from build123d import *

# Parameters (mm, degrees)
SKETCH_1_W               = 80
SKETCH_1_H               = 80
EXTRUDE_1_DEPTH          = 20
SKETCH_2_R               = 15
CUT_EXTRUDE_1_DEPTH      = 20
SKETCH_3_R               = 2
CUT_EXTRUDE_2_DEPTH      = 20
PATTERN_CIRCULAR_1_COUNT = 4
SKETCH_4_R               = 2.34
CUT_EXTRUDE_3_DEPTH      = 20
PATTERN_CIRCULAR_2_COUNT = 4
EXTRUDE_3_DEPTH          = 20
EXTRUDE_4_DEPTH          = 20
SKETCH_7_R               = 3
CUT_EXTRUDE_4_DEPTH      = 104.412342347
PATTERN_CIRCULAR_3_COUNT = 3


with BuildPart() as part:
    # 草图1 → 凸台-拉伸1 (new body)
    with BuildSketch(Plane.XY):
        Rectangle(SKETCH_1_W, SKETCH_1_H)
    extrude(amount=EXTRUDE_1_DEPTH)

    # 草图2 → 切除-拉伸1 (cut)
    with BuildSketch(Plane.XY.offset(20)):
        Circle(SKETCH_2_R)
    extrude(amount=-CUT_EXTRUDE_1_DEPTH, mode=Mode.SUBTRACT)

    # 草图3 → 切除-拉伸2 (cut)
    with BuildSketch(Plane.XY.offset(20)):
        with Locations((31, 31)):
            Circle(SKETCH_3_R)
    cut_extrude_2 = extrude(amount=-CUT_EXTRUDE_2_DEPTH, mode=Mode.SUBTRACT)

    # 阵列(圆周)1: 切除-拉伸2 ×4 about axis
    pattern_circular_1_axis = Axis((0, 0, 0), (0, 0, 1))
    for i in range(1, PATTERN_CIRCULAR_1_COUNT):
        add(cut_extrude_2.rotate(pattern_circular_1_axis, i * 360 / PATTERN_CIRCULAR_1_COUNT), mode=Mode.SUBTRACT)

    # 草图4 → 切除-拉伸3 (cut)
    with BuildSketch(Plane.XY.offset(20)):
        with Locations((16.24, 16.24)):
            Circle(SKETCH_4_R)
    cut_extrude_3 = extrude(amount=-CUT_EXTRUDE_3_DEPTH, mode=Mode.SUBTRACT)

    # 阵列(圆周)2: 切除-拉伸3 ×4 about axis
    pattern_circular_2_axis = Axis((0, 0, 0), (0, 0, 1))
    for i in range(1, PATTERN_CIRCULAR_2_COUNT):
        add(cut_extrude_3.rotate(pattern_circular_2_axis, i * 360 / PATTERN_CIRCULAR_2_COUNT), mode=Mode.SUBTRACT)

    # 草图5 → 凸台-拉伸3 (add)
    with BuildSketch(Plane(origin=(0, 0, 0), x_dir=(-1, 0, 0), z_dir=(0, 0, -1))):
        with BuildLine():
            Line((40, 40), (40, -40))
            ThreePointArc((40, -40), (52.262518595, -21.647844006), (56.568542495, 0))
            ThreePointArc((56.568542495, 0), (52.262518595, 21.647844006), (40, 40))
        make_face()
        with BuildLine():
            ThreePointArc((-40, -40), (0, -56.568542495), (40, -40))
            Line((40, -40), (-40, -40))
        make_face()
        with BuildLine():
            ThreePointArc((-40, 40), (-56.568542495, 0), (-40, -40))
            Line((-40, -40), (-40, 40))
        make_face()
        with BuildLine():
            Line((-40, 40), (40, 40))
            ThreePointArc((40, 40), (0, 56.568542495), (-40, 40))
        make_face()
    extrude(amount=-EXTRUDE_3_DEPTH)

    # 草图6 → 凸台-拉伸4 (add)
    with BuildSketch(Plane(origin=(0, 0, 0), x_dir=(-1, 0, 0), z_dir=(0, 0, -1))):
        with BuildLine():
            Line((76.568542495, 10), (55.677643628, 10))
            ThreePointArc((55.677643628, 10), (56.345377582, 5.019803303), (56.568542495, 0))
            ThreePointArc((56.568542495, 0), (56.345377582, -5.019803303), (55.677643628, -10))
            Line((55.677643628, -10), (76.568542495, -10))
            Line((76.568542495, -10), (76.568542495, 0))
            Line((76.568542495, 0), (76.568542495, 10))
        make_face()
    extrude_4 = extrude(amount=-EXTRUDE_4_DEPTH)

    # 草图7 → 切除-拉伸4 (cut, through all)
    with BuildSketch(Plane(origin=(0, -10, 0), x_dir=(-1, 0, 0), z_dir=(0, -1, 0))):
        with Locations(Location((66.123093062, -10, 0), (0, 0, 90))):
            Circle(SKETCH_7_R)
    cut_extrude_4 = extrude(amount=-CUT_EXTRUDE_4_DEPTH, mode=Mode.SUBTRACT)

    # 阵列(圆周)3: 凸台-拉伸4, 切除-拉伸4 ×3 about axis
    pattern_circular_3_axis = Axis((0, 0, 0), (0, 0, 1))
    add([extrude_4.rotate(pattern_circular_3_axis, i * 360 / PATTERN_CIRCULAR_3_COUNT) for i in range(1, PATTERN_CIRCULAR_3_COUNT)])
    add([cut_extrude_4.rotate(pattern_circular_3_axis, i * 360 / PATTERN_CIRCULAR_3_COUNT) for i in range(1, PATTERN_CIRCULAR_3_COUNT)], mode=Mode.SUBTRACT)


solid = part.part
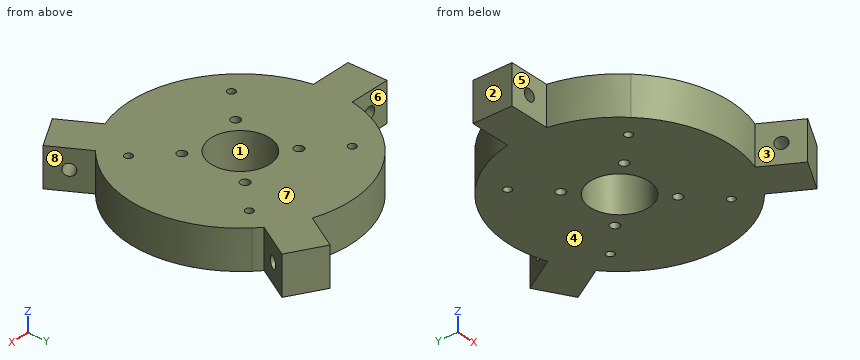
The model under review builds one solid part; all positions refer to its coordinate system, in mm. Face numbers are marked on the shaded views. A direction names the side the tool comes from. Give positions to 0.01 mm unless a question says otherwise; leave off trailing zeros. Order: outer loops, then holes, each group sorted by start corner. A loop starts at its lowest first (then second) coordinate and runs counter-clockwise, first axis right, second up. Notation, with made-up numbers: M -30,-11 L 24,-11 A27 cw 24,14 Z; hole C -27,36 d4. An arc over 180 degrees is marked long. Answer in a Markdown table with one row per item. Add a question column.
1. To check wall thickness, follow line 1 along Y through (x, z) = (31, 14.5); line 2 along X through (y, z) = (-5.5, 10); line 3 along X through (y, z) = (-17, 13). State the ranges of each line that lie inside material, in increasing order.
2. Add section A-A on z = 2.5. Count the separate pieces of the cut face and the enclosed holes in it, plus the area to 3 significant figures.
3. Machinability: for the marked faces 4, 5, 6, 7 and 8, which of the approach directions +Z, -Z, +X, -X, +Y, -Y give a long, thin tool a straight path to every point of the face, cutting with its end or side? Answer none if there is none.
4. For pin 1 Ø7 at (x, z) = (-66.12, 10) entering from +Y; pin 2 Ø5.5 at (x, y) = (16.24, 16.24) entering from +Z; pin 3 Ø4 at (x, z) = (-11, 9) entering from -Y; pin 4 Ø1.5 at (y, z) = (-32, 3.5) entering from +X, all flat-tipped, find the tip position at first contact; note any pin that passes through.
5. Add section C-C on y = 31. State the section outline as (x, z) points, plus the area to 3 significant figures.
6. Mouldability with a two-part tool opening along Y and no side actions: class the marked faces 1, 2 and 3 as released by +Y, released by -Y, zero draft, split by the parting line, or undercut.
7. Add section B-B on x = 0. State the section outline as (y, z) points.
The answers:
| question | item | result |
|---|---|---|
| 1 | line 1 | -70.52 to -33, -29 to 29, 33 to 70.52 |
| 1 | line 2 | -76.57 to -69.12, -63.12 to -13.96, 13.96 to 56.3 |
| 1 | line 3 | -53.95 to -18.45, -14.03 to 14.03, 18.45 to 53.95 |
| 2 | separate pieces | 1 |
| 2 | enclosed holes | 9 |
| 2 | area | 10,400 mm2 |
| 3 | face 4 | -Z, +X, -X, +Y, -Y |
| 3 | face 5 | +Z, -Z, -X, -Y |
| 3 | face 6 | +Z, -Z, -X, +Y |
| 3 | face 7 | +Z, +X, -X, +Y, -Y |
| 3 | face 8 | +Z, -Z, +X |
| 4 | pin 1 | y = 10 |
| 4 | pin 2 | z = 20 |
| 4 | pin 3 | y = -55.85 |
| 4 | pin 4 | x = 47.15 |
| 5 | outline | M -47.32,0 L -33,0 L -33,20 L -47.32,20 Z; M -29,0 L 29,0 L 29,20 L -29,20 Z; M 33,0 L 47.32,0 L 47.32,20 L 33,20 Z |
| 5 | area | 1,730 mm2 |
| 6 | face 1 | undercut |
| 6 | face 2 | zero draft |
| 6 | face 3 | released by -Y |
| 7 | outline | M -56.57,0 L -15,0 L -15,20 L -56.57,20 Z; M 15,0 L 56.57,0 L 56.57,20 L 15,20 Z |
